Part model, mm, in its own coordinate system. Round coordinates to 2 decimals unless told otherwise and drop trailing zeros. Write each loop counter-clockwise with the first axis right and the second up, starting at its lowest first coordinate (ties: lowest second). Pieces come first, ordered by that corner, then holes. Notation, with made-up numbers: M 82,31.5 L 128,31.5 A35 ccw 128,63.5 Z; hole C -11,71.5 d1. An arc over 180 degrees is marked long. Use one line per item in the form item = value. Start each with the question number.
Item 1: Cut at B-B, the plane y = -1. Give the cut face in (x, z).
Item 2: Flat gauge pins, fed straight in: pin 1 Ø1.5 at (x, z) = (96, 1) entering from +Y; pin 2 Ø1.5 at (y, z) = (19.5, 2) entering from +X; pin 3 Ø0.9 at (x, z) = (95, 1) entering from -Y. Where does each tip first touch, or does it go through?
Item 3: Cut at A-A, the plane z = 1.5. Give the cut face in (x, y), then the cut area to 3 significant figures.
Item 4: Cut at C-C, the plane y = 5.5. Give the cut face in (x, z), then the cut area to 3 significant figures.
Item 5: Probe L1, parallel to Y at x = 20.5, z = 0.7; L2, parallel to X at y = 16.5, z = 1.45; L3, parallel to X at y = 22, z = 2.9. List the from-to ranges inside material, lowest first.
from build123d import *

# Parameters (mm, degrees)
SALIENTE_EXTRUIR1_DEPTH = 3


with BuildPart() as part:
    # Model → Saliente-Extruir1 (new body)
    with BuildSketch(Plane.XY):
        with BuildLine():
            Line((96.785797009, 36.015840028), (93.785797009, 36.015840028))
            Line((93.785797009, 36.015840028), (93.785797009, 47.015840028))
            Line((93.785797009, 47.015840028), (31.751178944, 47.015840028))
            Line((31.751178944, 47.015840028), (29.260721948, 47.015840028))
            ThreePointArc((29.260721948, 47.015840028), (28.01691559, 46.383744396), (27.193529557, 45.257407597))
            ThreePointArc((27.193529557, 45.257407597), (23.155632663, 39.471985621), (16.34281865, 37.638605137))
            ThreePointArc((16.34281865, 37.638605137), (18.127374477, 28.444980745), (22.850598251, 20.358045222))
            ThreePointArc((22.850598251, 20.358045222), (19.57702332, 16.398637511), (14.878347932, 14.321222809))
            ThreePointArc((14.878347932, 14.321222809), (16.813155193, 8.973175992), (20.188286302, 4.395668604))
            ThreePointArc((20.188286302, 4.395668604), (17.693087489, 3.34861877), (15.188339451, 4.372614734))
            ThreePointArc((15.188339451, 4.372614734), (17.604909212, -2.266185371), (22.24359433, -7.594982292))
            ThreePointArc((22.24359433, -7.594982292), (19.566527855, -8.089682901), (16.920851616, -7.447958005))
            ThreePointArc((16.920851616, -7.447958005), (20.831880227, -11.496375144), (26.260721948, -12.984159972))
            Line((26.260721948, -12.984159972), (36.41114869, -12.984159972))
            Line((36.41114869, -12.984159972), (93.785797009, -12.984159972))
            Line((93.785797009, -12.984159972), (93.785797009, -1.984159972))
            Line((93.785797009, -1.984159972), (96.785797009, -1.984159972))
            Line((96.785797009, -1.984159972), (96.785797009, 8.015840028))
            Line((96.785797009, 8.015840028), (93.785797009, 8.015840028))
            Line((93.785797009, 8.015840028), (93.785797009, 26.015840028))
            Line((93.785797009, 26.015840028), (96.785797009, 26.015840028))
            Line((96.785797009, 26.015840028), (96.785797009, 36.015840028))
        make_face()
    extrude(amount=SALIENTE_EXTRUIR1_DEPTH)


solid = part.part
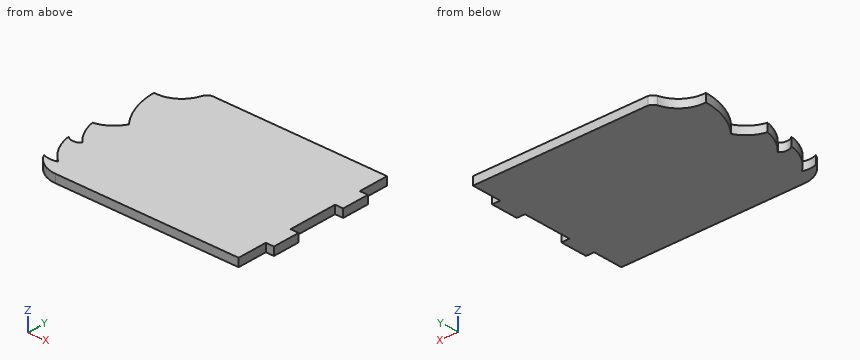
Model answer:
q1.outline = M 16.92,0 L 96.79,0 L 96.79,3 L 16.92,3 Z
q2.pin_1 = 36.02
q2.pin_2 = 93.79
q2.pin_3 = -1.98
q3.outline = M 14.88,14.32 A19.8 ccw 20.19,4.4 A3.54 cw 15.19,4.37 A19.35 ccw 22.24,-7.59 A6.52 cw 16.92,-7.45 A10.64 ccw 26.26,-12.98 L 93.79,-12.98 L 93.79,-1.98 L 96.79,-1.98 L 96.79,8.02 L 93.79,8.02 L 93.79,26.02 L 96.79,26.02 L 96.79,36.02 L 93.79,36.02 L 93.79,47.02 L 29.26,47.02 A3 ccw 27.19,45.26 A10.31 cw 16.34,37.64 A27.93 ccw 22.85,20.36 A11.18 cw Z
q3.area = 4,520 mm²
q4.outline = M 19.18,0 L 96.79,0 L 96.79,3 L 19.18,3 Z
q4.area = 233 mm²
q5.L1 = -11.29 to -8.05, -6.03 to 17.18, 23.62 to 38.13
q5.L2 = 19.71 to 93.79
q5.L3 = 21.58 to 93.79
